from build123d import *

# Parameters (mm, degrees)
SKETCH1_R           = 3.8
BOSS_EXTRUDE2_DEPTH = 3
SKETCH2_R           = 4.4
BOSS_EXTRUDE3_DEPTH = 25
CUT_EXTRUDE3_START  = -1
SKETCH10_R          = 4.4
CUT_EXTRUDE3_DEPTH  = 1
BOSS_EXTRUDE5_DEPTH = 3
SKETCH12_R          = 4.4
BOSS_EXTRUDE6_DEPTH = 5
SKETCH14_R          = 4.9
BOSS_EXTRUDE7_DEPTH = 1


with BuildPart() as part:
    # Sketch1 → Boss-Extrude2 (new body)
    with BuildSketch(Plane.XY):
        with BuildLine():
            Line((-48.125, 15.75), (48.125, 15.75))
            ThreePointArc((48.125, 15.75), (55.196067812, 12.821067812), (58.125, 5.75))
            Line((58.125, 5.75), (58.125, -15.75))
            Line((58.125, -15.75), (-58.125, -15.75))
            Line((-58.125, -15.75), (-58.125, 5.75))
            ThreePointArc((-58.125, 5.75), (-55.196067812, 12.821067812), (-48.125, 15.75))
        make_face()
        with Locations((31.875, -2.25)):
            Circle(SKETCH1_R, mode=Mode.SUBTRACT)
        with Locations((-31.875, 0.25)):
            Circle(SKETCH1_R, mode=Mode.SUBTRACT)
    extrude(amount=BOSS_EXTRUDE2_DEPTH)

    # Sketch2 → Boss-Extrude3 (add)
    with BuildSketch(Plane.XY.offset(3)):
        with Locations((8.725, 5.25)):
            Circle(SKETCH2_R)
        with Locations((-10.185, -4.75)):
            Circle(SKETCH2_R)
        with BuildLine():
            Line((55.625, 5.75), (55.625, -15.75))
            Line((55.625, -15.75), (58.125, -15.75))
            Line((58.125, -15.75), (58.125, 5.25))
            Line((58.125, 5.25), (58.125, 5.75))
            ThreePointArc((58.125, 5.75), (55.196067812, 12.821067812), (48.125, 15.75))
            Line((48.125, 15.75), (48.125, 13.25))
            ThreePointArc((48.125, 13.25), (53.428300859, 11.053300859), (55.625, 5.75))
        make_face()
        with BuildLine():
            Line((-58.125, -15.75), (-55.625, -15.75))
            Line((-55.625, -15.75), (-55.625, 5.75))
            ThreePointArc((-55.625, 5.75), (-53.428300859, 11.053300859), (-48.125, 13.25))
            Line((-48.125, 13.25), (-48.125, 15.75))
            ThreePointArc((-48.125, 15.75), (-55.196067812, 12.821067812), (-58.125, 5.75))
            Line((-58.125, 5.75), (-58.125, 5.25))
            Line((-58.125, 5.25), (-58.125, -15.75))
        make_face()
    extrude(amount=BOSS_EXTRUDE3_DEPTH)

    # Sketch10 → Cut-Extrude3 (cut)
    with BuildSketch(Plane.XY.offset(28).offset(CUT_EXTRUDE3_START)):
        with Locations((8.725, 5.25)):
            Circle(SKETCH10_R)
        with Locations((-10.185, -4.75)):
            Circle(SKETCH10_R)
    extrude(amount=CUT_EXTRUDE3_DEPTH, mode=Mode.SUBTRACT)

    # Sketch5 → Boss-Extrude5 (add)
    with BuildSketch(Plane.XY.offset(28)):
        with BuildLine():
            Line((-56.84687889, 3.934747007), (-56.975, -14.6))
            Line((-56.975, -14.6), (-55.625, -14.6))
            Line((-55.625, -14.6), (-55.625, 5.75))
            ThreePointArc((-55.625, 5.75), (-53.428300859, 11.053300859), (-48.125, 13.25))
            Line((-48.125, 13.25), (-48.125, 14.285189819))
            ThreePointArc((-48.125, 14.285189819), (-54.892622141, 11.137977782), (-56.84687889, 3.934747007))
        make_face()
        with BuildLine():
            Line((55.625, -14.6), (55.625, 5.75))
            ThreePointArc((55.625, 5.75), (53.428300859, 11.053300859), (48.125, 13.25))
            Line((48.125, 13.25), (48.125, 14.285189819))
            ThreePointArc((48.125, 14.285189819), (54.892622141, 11.137977782), (56.84687889, 3.934747007))
            Line((56.84687889, 3.934747007), (56.975, -14.6))
            Line((56.975, -14.6), (55.625, -14.6))
        make_face()
    extrude(amount=BOSS_EXTRUDE5_DEPTH)

    # Sketch12 → Boss-Extrude6 (add)
    with BuildSketch(Plane.XY.offset(27)):
        with Locations((-10.185, -4.75)):
            Circle(SKETCH12_R)
        with Locations((8.725, 5.25)):
            Circle(SKETCH12_R)
    extrude(amount=BOSS_EXTRUDE6_DEPTH)

    # Sketch14 → Boss-Extrude7 (add)
    with BuildSketch(Plane.XY.offset(15.5)):
        with Locations((-10.185, -4.75)):
            Circle(SKETCH14_R)
    extrude(amount=BOSS_EXTRUDE7_DEPTH)


solid = part.part
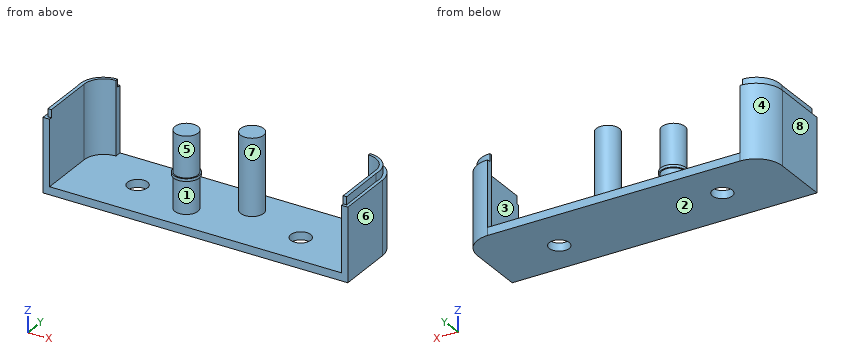
The model under review builds one solid part; all positions refer to its coordinate system, in mm. Face numbers are marked on the shaded views. A direction names the side the tool comes from. Coordinates: 2 decimals unless noted, no trailing zeros. Write each loop counter-clockwise with the first axis right and the second up, starting at its lowest first coordinate (ties: lowest second). Pieces come first, ordered by that corner, then holes. Notation, with made-up numbers: M 73,-17.75 L 101,-17.75 A16 ccw 101,-5.75 Z; hole C 68.5,33.5 d6. An arc over 180 degrees is marked long. Put each result on its own line as item: value.
1) Add section D-D on z = 6. Give the boundary of the cut face in (x, y) (3 decimals).
Computed:
outline: M -58.125,-15.75 L -55.625,-15.75 L -55.625,5.75 A7.5 cw -48.125,13.25 L -48.125,15.75 A10 ccw -58.125,5.75 Z; C -10.185,-4.75 d8.8; C 8.725,5.25 d8.8; M 48.125,13.25 A7.5 cw 55.625,5.75 L 55.625,-15.75 L 58.125,-15.75 L 58.125,5.75 A10 ccw 48.125,15.75 Z
2) Draft analysis for pull direction X (two halves, no side actions). For the marked faces 6, 7 and 8, state which applies: released by +X, released by -X, zero draft, split by the parting line, or undercut.
Computed:
face 6: released by +X
face 7: undercut
face 8: released by -X
3) Add section C-C on x = 34.5. Give the boundary of the cut face in (y, z), then the cut area to 3 significant figures.
Computed:
outline: M -15.75,0 L -5,0 L -5,3 L -15.75,3 Z; M 0.5,0 L 15.75,0 L 15.75,3 L 0.5,3 Z
area: 78.0 mm2
4) For the marked faces 1, 2, 3, 4 and 5, list the 3-axis set-ups (+Z, -Z, +X, -X, +Y, -Y) from which the entire face can be reached by the end or side of a thin tool; tool diameter is ignored.
Computed:
face 1: none
face 2: -Z, +X, -X, +Y, -Y
face 3: +Z, -Y
face 4: +Z, -Z, -X, +Y
face 5: +Z
5) Add section A-A on z = 30. Give the boundary of the cut face in (x, y) (3 decimals).
Computed:
outline: M -56.975,-14.6 L -55.625,-14.6 L -55.625,5.75 A7.5 cw -48.125,13.25 L -48.125,14.285 A8.85 ccw -56.847,3.935 Z; C -10.185,-4.75 d8.8; C 8.725,5.25 d8.8; M 48.125,13.25 A7.5 cw 55.625,5.75 L 55.625,-14.6 L 56.975,-14.6 L 56.847,3.935 A8.85 ccw 48.125,14.285 Z
6) Add section B-B on y = -2.25. State how many separate pieces and enclosed holes the cut face has, then the cut area to 3 significant figures.
Computed:
separate pieces: 3
enclosed holes: 0
area: 653 mm2
7) Clearance check with flat-ended pins moving along their axes: pin 1 Ø3 at (x, z) = (14, 5) entering from -Y; pin 2 Ø7 at (x, y) = (52.5, 3.5) entering from +Z; pin 3 Ø0.7 at (x, z) = (-56.5, 29.5) entering from -Y. State where each tip first meets the part, or that it passes through.
Computed:
pin 1: stops at y = 2.99
pin 2: stops at z = 31
pin 3: stops at y = -14.6
8) Wall thickness on probe 1 along X at (y, z) = (-5, 7) (3 decimals); probe 2 along X at (y, z) = (0.5, 7) (3 decimals); probe 3 along X at (y, z) = (3.5, 24) (3 decimals): over which ranges is each line inside the solid? List them lowest first. Write a range as [from, to].
Computed:
probe 1: x = [-58.125, -55.625], [-14.578, -5.792], [55.625, 58.125]
probe 2: x = [-58.125, -55.625], [55.625, 58.125]
probe 3: x = [-58.125, -55.625], [4.688, 12.762], [55.625, 58.125]
